```python
from build123d import *

# Parameters (mm, degrees)
ESQUISSE2_W             = 5.291502622
ESQUISSE2_H             = 1
ENL_V_MAT_EXTRU_1_DEPTH = 10
ESQUISSE3_R             = 1.5
FIXHOLES_DEPTH          = 3
REPEATFIXHOLES_COUNT    = 4


with BuildPart() as part:
    # Esquisse1 → MainRevolution (revolve)
    with BuildSketch(Plane.XY):
        Polygon((0, 0), (93.7, 0), (93.7, 4), (77.1, 4), (77.1, 9), (73.1, 9), (73.1, 15), (46, 15), (46, 13), (10, 13), (10, 12), (4, 12), (4, 2), (0, 2), align=None)
    revolve(axis=Axis((0, 0, 0), (1, 0, 0)))

    # Esquisse2 → Enl_v. mat.-Extru.1 (cut)
    with BuildSketch(Plane(origin=(93.7, 0, 0), x_dir=(0, 0, -1), z_dir=(1, 0, 0))):
        with Locations((0, 3.5)):
            Rectangle(ESQUISSE2_W, ESQUISSE2_H)
    extrude(amount=-ENL_V_MAT_EXTRU_1_DEPTH, mode=Mode.SUBTRACT)

    # Esquisse3 → FixHoles (cut)
    with BuildSketch(Plane(origin=(73.1, 0, 0), x_dir=(0, 0, -1), z_dir=(1, 0, 0))):
        with Locations((0, 13)):
            Circle(ESQUISSE3_R)
    fixholes = extrude(amount=-FIXHOLES_DEPTH, mode=Mode.SUBTRACT)

    # RepeatFixHoles: FixHoles ×4 about axis
    repeatfixholes_axis = Axis((0, 0, 0), (1, 0, 0))
    for i in range(1, REPEATFIXHOLES_COUNT):
        add(fixholes.rotate(repeatfixholes_axis, i * 360 / REPEATFIXHOLES_COUNT), mode=Mode.SUBTRACT)


solid = part.part
```
Here's how the part is built. I have some questions about the finished solid (model axes, mm). A direction names the side the tool comes from. Coordinates: 2 decimals unless noted, no trailing zeros. Loops run counter-clockwise (first coordinate to the right, second up) from the corner with the lowest first, then second, coordinate; pieces in that order, holes last. Notation, with made-up numbers: (12.5, -31) - (29.5, -31) arc R15 ccw to (29.5, -25) - close; hole circle Ø10 at (-27, 89.25). An arc over 180 degrees is marked (long way). Return JSON: item names as keys, results as strings. Group by question number.
Item 1: I need wall thicknesses on line 1 (X direction, y = 5, z = 2.75); line 2 (X direction, y = 7, z = 13); line 3 (Z direction, x = 72.45, y = -13). Which ranges of each line are inside material? Lowest first, please. Write a range as from..to.
Item 2: Will these pins go through, and if not, where does the flat tip stop? P1, Ø3.5, axis at y = 0, z = 13, coming from the -X side; P2, Ø2, axis at x = 68.5, y = 4.5, coming from the +Z side; P3, Ø2, axis at x = 15.5, y = 4, coming from the -Z side; P4, Ø5, axis at y = -1.5, z = -2.5, coming from the -X side.
Item 3: If we section it at D-D on y = 7.5: Write out the boundary of the cut face in (x, z), and give its area (3 significant figures).
Item 4: If we section it at C-C on x = 55.5: Write out the boundary of the cut face in (y, z).
Item 5: We'd pull the mould along Z, two halves only. Please class faces 1 (the face through (70.1, 0, -13)), 2 (the face through (59.36, -14.985, 0.66)), 3 (the face through (0, 0, 0)): +Z half, -Z half, draft (parallel to the pull), parting line (faces both ways), or undercut.
Item 6: On a 3-axis mill with a long thin cutter (end or side, diameter ignored), from which of +Z, -Z, +X, -X, +Y, -Y can I reach the whole of each face in a straight line? I mean faces 4 (the face through (93.7, 0, 0)), 5 (the face through (71.621, 1.386, 12.425)), 6 (the face through (89, 3, 0)), 7 (the face through (27.748, -10.316, -7.91)). Say none if no direction works.
Calculated:
{
 "1": {"line 1": "x = 4..77.1", "line 2": "x = 46..73.1", "line 3": "z = -7.48..-1.5, 1.5..7.48"},
 "2": {"P1": "stops at x = 4", "P2": "stops at z = 14.59", "P3": "stops at z = -12.65", "P4": "stops at x = 0"},
 "3": {"outline": "(4, -9.37) - (10, -9.37) - (10, -10.62) - (46, -10.62) - (46, -12.99) - (73.1, -12.99) - (73.1, -4.97) - (77.1, -4.97) - (77.1, 4.97) - (73.1, 4.97) - (73.1, 12.99) - (46, 12.99) - (46, 10.62) - (10, 10.62) - (10, 9.37) - (4, 9.37) - close", "area": "1,620 mm^2"},
 "4": {"outline": "circle Ø30 at (0, 0)"},
 "5": {"face 1": "undercut", "face 2": "parting line", "face 3": "draft"},
 "6": {"face 4": "+Z, -Z, +X, +Y, -Y", "face 5": "+X", "face 6": "+Z, -Z, +X, +Y", "face 7": "-X"}
}
